Read the model definition and answer for the solid it produces. Units are mm, in the model's axes. Coordinates: 2 decimals unless noted, no trailing zeros. Write each loop counter-clockwise with the first axis right and the second up, starting at its lowest first coordinate (ties: lowest second). Pieces come first, ordered by that corner, then holes.
Item 1: Each of these flat-tipped pins is pushed along its axis until it touches: P1, Ø3, axis at x = 7, z = -185, coming from the -Y side; P2, Ø4, axis at x = 5, z = -243.5, coming from the +Y side; P3, Ø4, axis at x = 8.5, z = -180, coming from the +Y side; P4, Ø11.5, axis at y = 150.81, z = -136.72, coming from the -X side. Where does it stop, or does it pass through?
Item 2: Straight lines are drawn through the part: probe 1 along Y at (x, z) = (12, -102.5); probe 2 along Z at (x, y) = (9.25, 120); probe 3 along Y at (x, z) = (10.75, -131). For each, find the intervals that lie inside material, in ascending order.
Item 3: Section C-C (y = 13) is taken. Give the vertices of the cut face in (x, z).
Item 4: Section B-B (z = -202) is taken. Give the vertices of the cut face in (x, y), then the cut area to 3 significant figures.
from build123d import *

# Parameters (mm, degrees)
MAIN_DEPTH  = 12.7
SKETCH2_W   = 12.7
SKETCH2_H   = 63.5
STAND_DEPTH = 68.2625
SKETCH3_R   = 6.35
AXLE_DEPTH  = 12.7
FILLET1_R   = 31.75
FILLET2_R   = 31.75


with BuildPart() as part:
    # Sketch1 → main (new body)
    with BuildSketch(Plane(origin=(0, 0, 0), x_dir=(0, 0, -1), z_dir=(1, 0, 0))):
        Polygon((0, 0), (298.45, 0), (184.15, 114.3), (0, 114.3), align=None)
    extrude(amount=MAIN_DEPTH)

    # Sketch2 → stand (add)
    with BuildSketch(Plane(origin=(0, 114.3, 0), x_dir=(1, 0, 0), z_dir=(0, 1, 0))):
        with Locations((6.35, 136.71804)):
            Rectangle(SKETCH2_W, SKETCH2_H)
    extrude(amount=STAND_DEPTH)

    # Sketch3 → axle (cut)
    with BuildSketch(Plane(origin=(12.7, 0, 0), x_dir=(0, 0, -1), z_dir=(1, 0, 0))):
        with Locations((136.71804, 150.8125)):
            Circle(SKETCH3_R)
    extrude(amount=-AXLE_DEPTH, mode=Mode.SUBTRACT)

    # Fillet1
    fillet1_edges = [part.edges().sort_by_distance(p)[0] for p in [
        (6.35, 182.5625, -168.46804),
    ]]
    fillet(fillet1_edges, radius=FILLET1_R)

    # Fillet2
    fillet2_edges = [part.edges().sort_by_distance(p)[0] for p in [
        (6.35, 182.5625, -104.96804),
    ]]
    fillet(fillet2_edges, radius=FILLET2_R - 0.0001)  # a hair under: the kernel refuses the full size


solid = part.part
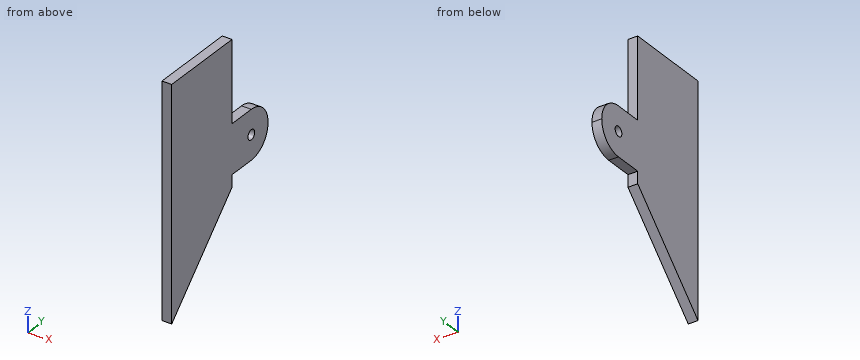
Established:
1. P1: stops at y = 0
1. P2: stops at y = 56.95
1. P3: stops at y = 114.3
1. P4: passes through
2. probe 1: y = 0 to 114.3
2. probe 2: z = -168.47 to -104.97
2. probe 3: y = 0 to 148.05, 153.57 to 182.04
3. outline: (0, -285.45) - (12.7, -285.45) - (12.7, 0) - (0, 0) - close
4. outline: (0, 0) - (12.7, 0) - (12.7, 96.45) - (0, 96.45) - close
4. area: 1,220 mm2
